from build123d import *

# Parameters (mm, degrees)
BOSS_EXTRUDE1_DEPTH                               = 6
CSK_FOR_8_FLAT_HEAD_MACHINE_SCREW_100_D           = 4.3053
CSK_FOR_8_FLAT_HEAD_MACHINE_SCREW_100_CSINK_D     = 8.4328
CSK_FOR_8_FLAT_HEAD_MACHINE_SCREW_100_CSINK_ANGLE = 100
SKETCH5_R                                         = 1.905
BOSS_EXTRUDE2_DEPTH                               = 2.5


with BuildPart() as part:
    # Sketch1 → Boss-Extrude1 (new body)
    with BuildSketch(Plane.XY):
        with BuildLine():
            Line((-26.167728216, 59.5), (26.167728216, 59.5))
            ThreePointArc((26.167728216, 59.5), (65, 0), (26.167728216, -59.5))
            Line((26.167728216, -59.5), (-26.167728216, -59.5))
            ThreePointArc((-26.167728216, -59.5), (-65, 0), (-26.167728216, 59.5))
        make_face()
        with BuildLine():
            Line((-23.650581388, 48.1), (23.650581388, 48.1))
            ThreePointArc((23.650581388, 48.1), (53.6, 0), (23.650581388, -48.1))
            Line((23.650581388, -48.1), (-23.650581388, -48.1))
            ThreePointArc((-23.650581388, -48.1), (-53.6, 0), (-23.650581388, 48.1))
        make_face(mode=Mode.SUBTRACT)
    extrude(amount=BOSS_EXTRUDE1_DEPTH)

    # CSK for #8 Flat Head Machine Screw (100)1 (through all)
    with Locations(Plane.XY.offset(6)):
        with Locations((0, 0), (41.985, 41.985), (-41.985, -41.985), (-41.985, 41.985), (41.985, -41.985)):
            CounterSinkHole(CSK_FOR_8_FLAT_HEAD_MACHINE_SCREW_100_D / 2, CSK_FOR_8_FLAT_HEAD_MACHINE_SCREW_100_CSINK_D / 2, counter_sink_angle=CSK_FOR_8_FLAT_HEAD_MACHINE_SCREW_100_CSINK_ANGLE)

    # Sketch5 → Boss-Extrude2 (add)
    with BuildSketch(Plane(origin=(0, 0, 0), x_dir=(-1, 0, 0), z_dir=(0, 0, -1))):
        with Locations(Location((-59.2455, 0, 0), (0, 0, 180))):
            Circle(SKETCH5_R)
        with Locations(Location((59.2455, 0, 0), (0, 0, 180))):
            Circle(SKETCH5_R)
    extrude(amount=BOSS_EXTRUDE2_DEPTH)


solid = part.part
CAD build for the part. Positions are in the model's coordinates, mm. A direction names the side the tool comes from. Coordinates: 2 decimals unless noted, no trailing zeros. Order: outer loops, then holes, each group sorted by start corner. A loop starts at its lowest first (then second) coordinate and runs counter-clockwise, first axis right, second up.
Item 1: Drill centre lines: L1, parallel to X at y = -1, z = 2.75; L2, parallel to Y at x = 8, z = 5.25; L3, parallel to X at y = 19, z = 3. Where is each one in solid material? Low to high.
Check sheet entries:
L1: x = -64.99 to -53.59, 53.59 to 64.99
L2: y = -59.5 to -48.1, 48.1 to 59.5
L3: x = -62.16 to -50.12, 50.12 to 62.16
Item 2: Pin check, flat tips, straight feed: pin 1 Ø5.5 at (x, y) = (-41.985, 41.985) entering from -Z; pin 2 Ø2.5 at (x, y) = (41.985, -41.985) entering from -Z; pin 3 Ø5 at (x, z) = (-44, 1.5) entering from +Y; pin 4 Ø5 at (x, y) = (41.985, 41.985) entering from +Z. Stop position of each tip, or through.
Check sheet entries:
pin 1: stops at z = 0
pin 2: passes through
pin 3: stops at y = 50.03
pin 4: stops at z = 4.56
Item 3: Band-saw the part on D-D on y = -24.5. List the corners of the cut face in (x, z), plus the area to 3 significant figures.
Check sheet entries:
outline: (-60.21, 0) - (-47.67, 0) - (-47.67, 6) - (-60.21, 6) - close; (47.67, 0) - (60.21, 0) - (60.21, 6) - (47.67, 6) - close
area: 150 mm2
Item 4: Two-plate mould, pull along X, no slides. Class faces 1 (the face through (-64.99, -1.05, 2.96)), 2 (the face through (-59, 0, -2.5)), 3 (the face through (-39.834, -41.89, 2.104)): +X half, -X half, draft (parallel to the pull), parting line (faces both ways), or undercut.
Check sheet entries:
face 1: -X half
face 2: draft
face 3: undercut
Item 5: Band-saw the part on B-B on y = 0. List the corners of the cut face in (x, z), plus the area to 3 significant figures.
Check sheet entries:
outline: (-65, 0) - (-61.15, 0) - (-61.15, -2.5) - (-57.34, -2.5) - (-57.34, 0) - (-53.6, 0) - (-53.6, 6) - (-65, 6) - close; (53.6, 0) - (57.34, 0) - (57.34, -2.5) - (61.15, -2.5) - (61.15, 0) - (65, 0) - (65, 6) - (53.6, 6) - close
area: 156 mm2
Item 6: 3-axis set-ups, long thin cutter, end or side, ignore diameter. For faces 4 (the face through (0, -48.1, 3)), 5 (the face through (64.99, 1.05, 2.96)): which of +Z, -Z, +X, -X, +Y, -Y reach the whole face in a straight line?
Check sheet entries:
face 4: +Z, -Z
face 5: +Z, -Z, +X
Item 7: Band-saw the part on C-C on z = 1.75. List the corners of the cut face in (x, y) (3 decimals).
Check sheet entries:
outline: (-26.168, -59.5) - (26.168, -59.5) arc R65 ccw to (26.168, 59.5) - (-26.168, 59.5) arc R65 ccw to start; hole circle Ø4.305 at (-41.985, -41.985); hole circle Ø4.305 at (-41.985, 41.985); hole (-23.651, -48.1) - (23.651, -48.1) arc R53.6 ccw to (23.651, 48.1) - (-23.651, 48.1) arc R53.6 ccw to start; hole circle Ø4.305 at (41.985, -41.985); hole circle Ø4.305 at (41.985, 41.985)
Item 8: Band-saw the part on A-A on x = -1.5. List the corners of the cut face in (y, z), plus the area to 3 significant figures.
Check sheet entries:
outline: (-59.5, 0) - (-48.1, 0) - (-48.1, 6) - (-59.5, 6) - close; (48.1, 0) - (59.5, 0) - (59.5, 6) - (48.1, 6) - close
area: 137 mm2
